from build123d import *

# Parameters (mm, degrees)
SKETCH1_R           = 3.475
BOSS_EXTRUDE1_DEPTH = 2
SKETCH2_R           = 1.575
CUT_EXTRUDE1_DEPTH  = 27.009613607
SKETCH3_W           = 3.796627216
SKETCH3_H           = 5.505702191
CUT_EXTRUDE2_DEPTH  = 27.009613607


with BuildPart() as part:
    # Sketch1 → Boss-Extrude1 (new body)
    with BuildSketch(Plane(origin=(0, 0, 0), x_dir=(1, 0, 0), z_dir=(0, 1, 0))):
        with BuildLine():
            Line((-19.5, -14.5), (19.5, -14.5))
            ThreePointArc((19.5, -14.5), (20.914213562, -13.914213562), (21.5, -12.5))
            Line((21.5, -12.5), (21.5, 12.5))
            ThreePointArc((21.5, 12.5), (20.914213562, 13.914213562), (19.5, 14.5))
            Line((19.5, 14.5), (-19.5, 14.5))
            ThreePointArc((-19.5, 14.5), (-20.914213562, 13.914213562), (-21.5, 12.5))
            Line((-21.5, 12.5), (-21.5, -12.5))
            ThreePointArc((-21.5, -12.5), (-20.914213562, -13.914213562), (-19.5, -14.5))
        make_face()
        with Locations(Location((-16.77, 0, 0), (0, 0, 270))):
            Circle(SKETCH1_R, mode=Mode.SUBTRACT)
        with Locations(Location((16.77, 0, 0), (0, 0, 270))):
            Circle(SKETCH1_R, mode=Mode.SUBTRACT)
        with BuildLine():
            Line((-7.5, -9.5), (7.5, -9.5))
            ThreePointArc((7.5, -9.5), (8.914213562, -8.914213562), (9.5, -7.5))
            Line((9.5, -7.5), (9.5, 7.5))
            ThreePointArc((9.5, 7.5), (8.914213562, 8.914213562), (7.5, 9.5))
            Line((7.5, 9.5), (-7.5, 9.5))
            ThreePointArc((-7.5, 9.5), (-8.914213562, 8.914213562), (-9.5, 7.5))
            Line((-9.5, 7.5), (-9.5, -7.5))
            ThreePointArc((-9.5, -7.5), (-8.914213562, -8.914213562), (-7.5, -9.5))
        make_face(mode=Mode.SUBTRACT)
    extrude(amount=BOSS_EXTRUDE1_DEPTH)

    # Sketch2 → Cut-Extrude1 (cut, through all)
    with BuildSketch(Plane(origin=(0, 2, 0), x_dir=(1, 0, 0), z_dir=(0, 1, 0))):
        with Locations(Location((0, 11.63, 0), (0, 0, 270))):
            Circle(SKETCH2_R)
    extrude(amount=-CUT_EXTRUDE1_DEPTH, mode=Mode.SUBTRACT)

    # Sketch3 → Cut-Extrude2 (cut, through all)
    with BuildSketch(Plane(origin=(0, 2, 0), x_dir=(1, 0, 0), z_dir=(0, 1, 0))):
        with Locations((6.026686392, -11.747148905)):
            Rectangle(SKETCH3_W, SKETCH3_H)
    extrude(amount=-CUT_EXTRUDE2_DEPTH, mode=Mode.SUBTRACT)


solid = part.part
The listing builds one solid part. Answer for the finished solid, in the listing's coordinates (mm). A direction names the side the tool comes from. Give positions to 0.01 mm unless a question says otherwise; leave off trailing zeros. Write each loop counter-clockwise with the first axis right and the second up, starting at its lowest first coordinate (ties: lowest second). Pieces come first, ordered by that corner, then holes.
1) Section D-D (y = 1.4) is taken. Write down the section's boundary in (x, z) (3 decimals), and give its area (3 significant figures).
2) Section A-A (x = 0) is taken. Write down the section's boundary in (y, z) (3 decimals), and give its area (3 significant figures).
3) For a pull along Z with two mould halves and no side action, classify faces 1 (the face through (-8.93, 0.99, 8.9)), 2 (the face through (9.5, 1, 0)), 3 (the face through (-10, 0, 0)), 4 (the face through (14, 1, 14.5)) as pulls with the +Z half, pulls with the -Z half, needs draft (parallel to the pull), parting line crosses it, or undercut.
4) Find the intervals of material crossed by L1, parallel to X at y = 0.85, z = 0 (3 decimals); L2, parallel to Z at x = -2, y = 1.75; L3, parallel to X at y = 1, z = -3.75, in increasing order.
5) A tool of negligible diameter and unlimited length cuts with its end or side. For faces 5 (the face through (-20.93, 0.99, 13.9)), 6 (the face through (9.045, 0.986, 8.77)), 7 (the face through (4.128, 1, 12)), from which of +Z, -Z, +X, -X, +Y, -Y can it reach the whole face along a straight path? Write none if from no direction.
6) Section C-C (z = 0) is taken. Write down the section's boundary in (x, y) (3 decimals).
7) Section B-B (z = -4.5) is taken. Write down the section's boundary in (x, y), and give its area (3 significant figures).
Response:
1. outline: (-21.5, -12.5) arc R2 ccw to (-19.5, -14.5) - (19.5, -14.5) arc R2 ccw to (21.5, -12.5) - (21.5, 12.5) arc R2 ccw to (19.5, 14.5) - (7.925, 14.5) - (7.925, 9.454) arc R2 cw to (9.5, 7.5) - (9.5, -7.5) arc R2 cw to (7.5, -9.5) - (-7.5, -9.5) arc R2 cw to (-9.5, -7.5) - (-9.5, 7.5) arc R2 cw to (-7.5, 9.5) - (4.128, 9.5) - (4.128, 14.5) - (-19.5, 14.5) arc R2 ccw to (-21.5, 12.5) - close; hole circle Ø6.95 at (-16.77, 0); hole circle Ø3.15 at (0, -11.63); hole circle Ø6.95 at (16.77, 0)
1. area: 783 mm2
2. outline: (0, -14.5) - (2, -14.5) - (2, -13.205) - (0, -13.205) - close; (0, -10.055) - (2, -10.055) - (2, -9.5) - (0, -9.5) - close; (0, 9.5) - (2, 9.5) - (2, 14.5) - (0, 14.5) - close
2. area: 13.7 mm2
3. face 1: undercut
3. face 2: undercut
3. face 3: needs draft
3. face 4: pulls with the +Z half
4. L1: x = -21.5 to -20.245, -13.295 to -9.5, 9.5 to 13.295, 20.245 to 21.5
4. L2: z = -14.5 to -9.5, 9.5 to 14.5
4. L3: x = -21.5 to -9.5, 9.5 to 21.5
5. face 5: +Z, -X, +Y, -Y
5. face 6: +Y, -Y
5. face 7: +Z, +Y, -Y
6. outline: (-21.5, 0) - (-20.245, 0) - (-20.245, 2) - (-21.5, 2) - close; (-13.295, 0) - (-9.5, 0) - (-9.5, 2) - (-13.295, 2) - close; (9.5, 0) - (13.295, 0) - (13.295, 2) - (9.5, 2) - close; (20.245, 0) - (21.5, 0) - (21.5, 2) - (20.245, 2) - close
7. outline: (-21.5, 0) - (-9.5, 0) - (-9.5, 2) - (-21.5, 2) - close; (9.5, 0) - (21.5, 0) - (21.5, 2) - (9.5, 2) - close
7. area: 48.0 mm2
